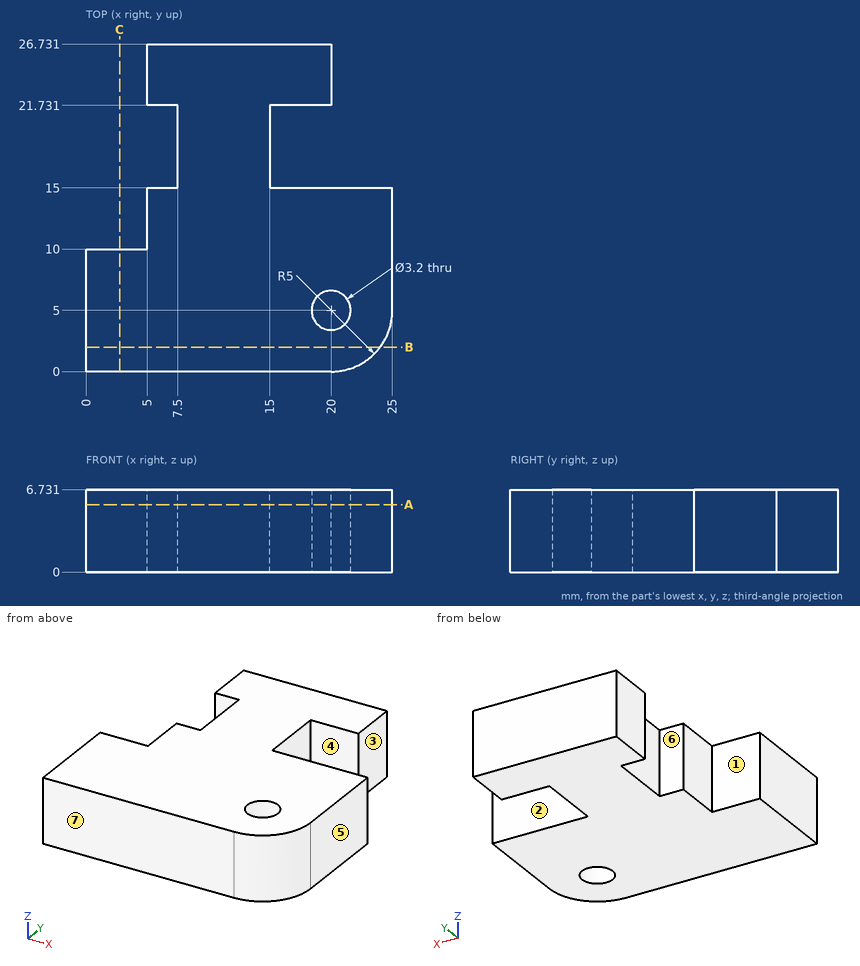
Design review of the part shown in the three views and the two pictorial views. Dimensions are in mm from the part's minimum x, y and z. A direction names the side the tool comes from. Coordinates: 2 decimals unless noted, no trailing zeros. Loops run counter-clockwise (first coordinate to the right, second up) from the corner with the lowest first, then second, coordinate; pieces in that order, holes last. Notation, with made-up numbers: M 54,-34.5 L 90,-34.5 A19 ccw 90,-16.5 Z; hole C -39,50 d10. An arc over 180 degrees is marked long. Put each result on its own line as item: value. Start each with the question number.
Q1. Add section B-B (y = 2). Write out the cut boundary in (x, z), and give its area (3 significant figures).
Q2. Add section C-C (x = 2.75). Write out the cut boundary in (y, z).
Q3. Wall thickness on line 1 (Y direction, x = 6.75, z = 2.25); line 2 (X direction, y = 13, z = 6); line 3 (X direction, y = 24, z = 5): over which ranges is each line inside the solid? List them lowest first.
Q4. The part is to be moulded in two halves that separate along Y. For the marked faces 4, 5, 6 and 7, say which applies: +Y half, -Y half, draft (parallel to the pull), parting line (faces both ways), or undercut.
Q5. Clearance check with flat-ended pins moving along their axes: pin 1 (1.5 mm diameter, centred on y = 14.5, z = 2, fed in from -X); pin 2 (1.5 mm diameter, centred on y = 25, z = 5, fed in from +X); pin 3 (2.5 mm diameter, centred on x = 2, z = 2, fed in from +Y). State where each tip first meets the part, or that it passes through.
Q6. Add section A-A (z = 5.5). Write out the cut boundary in (x, y), and give its area (3 significant figures).
Q7. For the marked faces 1, 2 and 3, list the 3-axis set-ups (+Z, -Z, +X, -X, +Y, -Y) from which the entire face can be reached by the end or side of a thin tool; tool diameter is ignored.
Answers:
1. outline: M 0,0 L 24,0 L 24,6.73 L 0,6.73 Z
1. area: 162 mm^2
2. outline: M 0,0 L 10,0 L 10,6.73 L 0,6.73 Z
3. line 1: y = 0 to 15, 21.73 to 26.73
3. line 2: x = 5 to 25
3. line 3: x = 5 to 20
4. face 4: undercut
4. face 5: draft
4. face 6: undercut
4. face 7: -Y half
5. pin 1: stops at x = 5
5. pin 2: stops at x = 20
5. pin 3: stops at y = 10
6. outline: M 0,0 L 20,0 A5 ccw 25,5 L 25,15 L 15,15 L 15,21.73 L 20,21.73 L 20,26.73 L 5,26.73 L 5,21.73 L 7.5,21.73 L 7.5,15 L 5,15 L 5,10 L 0,10 Z; hole C 20,5 d3.2
6. area: 462 mm^2
7. face 1: +Z, -Z, -X, +Y
7. face 2: +Z, -Z, +X
7. face 3: +Z, -Z, +X, +Y
